CAD build for the part. Positions are in the model's coordinates, mm. Face numbers are marked on the shaded views. A direction names the side the tool comes from. Round coordinates to 2 decimals unless told otherwise and drop trailing zeros. Write each loop counter-clockwise with the first axis right and the second up, starting at its lowest first coordinate (ties: lowest second). Pieces come first, ordered by that corner, then holes. Notation, with made-up numbers: (-9, 15) - (27, 15) arc R12 ccw to (27, 27) - close; hole circle Ø3 at (27.25, 85.25). An arc over 180 degrees is marked (long way). Use one line per item in the form item = value. Start each with the question number.
Item 1: Band-saw the part on D-D, the plane z = -89. List the corners of the cut face in (x, y) (3 decimals), and give its area (3 significant figures).
Item 2: Band-saw the part on B-B, the plane y = 37.5. List the corners of the cut face in (x, z) (3 decimals), and give its area (3 significant figures).
Item 3: Pull direction Z, two halves, no side cores. Call the marked faces 3, 4 and 5: +Z half, -Z half, draft (parallel to the pull), parting line (faces both ways), or undercut.
Item 4: Band-saw the part on C-C, the plane x = -46.5. List the corners of the cut face in (y, z) (3 decimals).
Item 5: Pin check, flat tips, straight feed: pin 1 (12 mm diameter, centred on x = -41, z = 43.5, fed in from +Y) (3 decimals); pin 2 (3 mm diameter, centred on x = -69, z = 93.5, fed in from +Y). Stop position of each tip, or through.
Item 6: Tool access for the marked faces 1 and 2: list every direction of +Z, -Z, +X, -X, +Y, -Y with a clear straight run to the whole face (end or side of a thin tool).
Item 7: Band-saw the part on A-A, the plane z = 62.5. List the corners of the cut face in (x, y) (3 decimals).
Item 8: Drill centre lines: L1, parallel to X at y = 36, z = -87 (3 decimals); L2, parallel to Z at x = -82, y = 7.5 (3 decimals); L3, parallel to Y at x = 79.5, z = 85.5 (3 decimals). Where is each one in solid material? Low to high.
from build123d import *

# Parameters (mm, degrees)
SKETCH1_W           = 184.15
SKETCH1_H           = 214.63
BOSS_EXTRUDE1_DEPTH = 47.625
SHELL1_T            = -3.175
BOSS_EXTRUDE2_DEPTH = 5.953125


with BuildPart() as part:
    # Sketch1 → Boss-Extrude1 (new body)
    with BuildSketch(Plane(origin=(0, 0, 0), x_dir=(1, 0, 0), z_dir=(0, 1, 0))):
        Rectangle(SKETCH1_W, SKETCH1_H)
    extrude(amount=BOSS_EXTRUDE1_DEPTH)

    # Shell1
    shell1_openings = [part.faces().sort_by_distance(p)[0] for p in [
        (0, 47.625, 0),
    ]]
    offset(amount=SHELL1_T, openings=shell1_openings, kind=Kind.INTERSECTION)

    # Sketch3 → Boss-Extrude2 (add)
    with BuildSketch(Plane(origin=(0, 3.175, 0), x_dir=(1, 0, 0), z_dir=(0, 1, 0))):
        Polygon((-27.597261314, -91.44), (-24.847630657, -96.2025), (-19.348369343, -96.2025), (-16.598738686, -91.44), (-19.348369343, -86.6775), (-24.847630657, -86.6775), align=None)
        Polygon((-71.793261314, -91.44), (-69.043630657, -96.2025), (-63.544369343, -96.2025), (-60.794738686, -91.44), (-63.544369343, -86.6775), (-69.043630657, -86.6775), align=None)
        Polygon((16.598738686, -91.44), (19.348369343, -96.2025), (24.847630657, -96.2025), (27.597261314, -91.44), (24.847630657, -86.6775), (19.348369343, -86.6775), align=None)
        Polygon((60.794738686, -91.44), (63.544369343, -96.2025), (69.043630657, -96.2025), (71.793261314, -91.44), (69.043630657, -86.6775), (63.544369343, -86.6775), align=None)
        Polygon((-27.597261314, 91.44), (-24.847630657, 86.6775), (-19.348369343, 86.6775), (-16.598738686, 91.44), (-19.348369343, 96.2025), (-24.847630657, 96.2025), align=None)
        Polygon((16.598738686, 91.44), (19.348369343, 86.6775), (24.847630657, 86.6775), (27.597261314, 91.44), (24.847630657, 96.2025), (19.348369343, 96.2025), align=None)
        Polygon((60.794738686, 91.44), (63.544369343, 86.6775), (69.043630657, 86.6775), (71.793261314, 91.44), (69.043630657, 96.2025), (63.544369343, 96.2025), align=None)
        Polygon((-71.793261314, 91.44), (-69.043630657, 86.6775), (-63.544369343, 86.6775), (-60.794738686, 91.44), (-63.544369343, 96.2025), (-69.043630657, 96.2025), align=None)
    extrude(amount=BOSS_EXTRUDE2_DEPTH)


solid = part.part
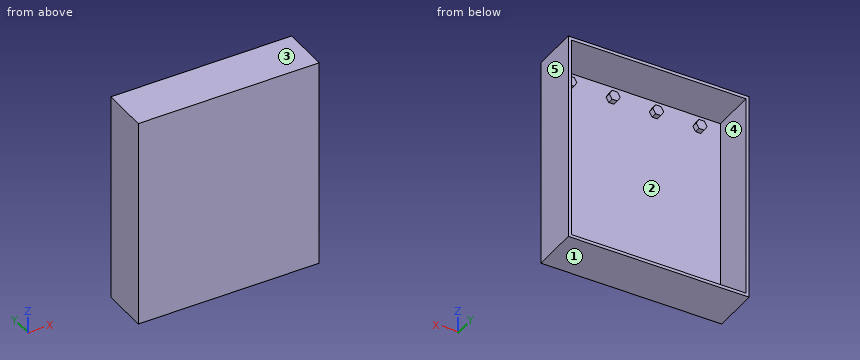
Determined:
q1.outline = (-92.075, 0) - (92.075, 0) - (92.075, 47.625) - (88.9, 47.625) - (88.9, 3.175) - (70.385, 3.175) - (70.385, 9.128) - (62.203, 9.128) - (62.203, 3.175) - (26.189, 3.175) - (26.189, 9.128) - (18.007, 9.128) - (18.007, 3.175) - (-18.007, 3.175) - (-18.007, 9.128) - (-26.189, 9.128) - (-26.189, 3.175) - (-62.203, 3.175) - (-62.203, 9.128) - (-70.385, 9.128) - (-70.385, 3.175) - (-88.9, 3.175) - (-88.9, 47.625) - (-92.075, 47.625) - close
q1.area = 1,060 mm²
q2.outline = (-92.075, -107.315) - (92.075, -107.315) - (92.075, 107.315) - (-92.075, 107.315) - close; hole (-88.9, -104.14) - (88.9, -104.14) - (88.9, 104.14) - (-88.9, 104.14) - close
q2.area = 2,490 mm²
q3.face_3 = +Z half
q3.face_4 = undercut
q3.face_5 = draft
q4.outline = (0, -107.315) - (47.625, -107.315) - (47.625, -104.14) - (3.175, -104.14) - (3.175, 104.14) - (47.625, 104.14) - (47.625, 107.315) - (0, 107.315) - close
q5.pin_1 = 3.175
q5.pin_2 = 9.13
q6.face_1 = -Z, +X, -X, +Y, -Y
q6.face_2 = +Y
q7.outline = (-92.075, 0) - (92.075, 0) - (92.075, 47.625) - (88.9, 47.625) - (88.9, 3.175) - (-88.9, 3.175) - (-88.9, 47.625) - (-92.075, 47.625) - close
q8.L1 = -92.075 to -88.9, 88.9 to 92.075
q8.L2 = -107.315 to -104.14, 104.14 to 107.315
q8.L3 = 0 to 3.175
